```python
from build123d import *

# Parameters (mm, degrees)
F1_DEPTH = 50
F0_W     = 5
F0_H     = 13.255382
F2_DEPTH = 68
F3_R     = 2.6
F4_DEPTH = 9.584522
F5_R     = 5.083522
F6_DEPTH = 48


with BuildPart() as f1:
    # F0 (on Top) → F1 (new body)
    with BuildSketch(Plane.XY):
        with BuildLine():
            ThreePointArc((2.5, -6.627691), (5.826023, -4.029111), (7.083522, 0))
            ThreePointArc((7.083522, 0), (5.826023, 4.029111), (2.5, 6.627691))
            Line((2.5, 6.627691), (2.5, -6.627691))
        make_face()
        with BuildLine():
            Line((-2.5, 6.627691), (2.5, 6.627691))
            ThreePointArc((2.5, 6.627691), (0, 7.083522), (-2.5, 6.627691))
        make_face()
        with BuildLine():
            ThreePointArc((-2.5, -6.627691), (0, -7.083522), (2.5, -6.627691))
            Line((2.5, -6.627691), (-2.5, -6.627691))
        make_face()
        with BuildLine():
            Line((-2.5, -6.627691), (-2.5, 6.627691))
            ThreePointArc((-2.5, 6.627691), (-7.083522, 0), (-2.5, -6.627691))
        make_face()
    extrude(amount=F1_DEPTH)

    # F0 (on Top) → F2 (join)
    with BuildSketch(Plane.XY):
        Rectangle(F0_W, F0_H)
    extrude(amount=F2_DEPTH)

    # F3 (on face) → F4 (cut, through all)
    with BuildSketch(Plane.YZ.offset(2.5)):
        with Locations((0, 60)):
            Circle(F3_R)
    extrude(amount=-F4_DEPTH, mode=Mode.SUBTRACT)

    # F5 (on face) → F6 (cut)
    with BuildSketch(Plane(origin=(0, 0, 0), x_dir=(1, 0, 0), z_dir=(0, 0, -1))):
        Circle(F5_R)
    extrude(amount=-F6_DEPTH, mode=Mode.SUBTRACT)


solid = f1.part
```
Design review of the part built by this model. Coordinates are the model's own, in mm. A direction names the side the tool comes from. Give positions to 0.01 mm unless a question says otherwise; leave off trailing zeros. Loops run counter-clockwise (first coordinate to the right, second up) from the corner with the lowest first, then second, coordinate; pieces in that order, holes last. Notation, with made-up numbers: M -33.75,1.25 L -19.75,1.25 A30 ccw -19.75,24.25 Z; hole C 52.5,-28.75 d7. An arc over 180 degrees is marked long. Return JSON: item names as keys, results as strings. Group by question number.
Item 1: Insertion check: pin 1 Ø1.4 at (x, y) = (4.5, 0) entering from +Z; pin 2 Ø4 at (y, z) = (3, 48.5) entering from -X; pin 3 Ø5 at (x, z) = (-4.5, 44) entering from -Y. Each pin has a flat end and moves straight along its axis. Give the tip position at first contact, or say it passes through.
Item 2: We need section D-D (x = 4). Give the boundary of the cut face in (y, z).
Item 3: We need section B-B (x = -0.25). Give the boundary of the cut face in (y, z).
Item 4: For probe 1 along Y at (x, z) = (0, 37); probe 2 along X at (y, z) = (-2, 64), list the stretches that pass through material, from the lowest coordinate up.
Item 5: We need section C-C (z = 6). Give the boundary of the cut face in (x, y).
Item 6: We need section A-A (z = 60). Give the boundary of the cut face in (x, y).
Item 7: Mouldability with a two-part tool opening along Y and no side actions: class faces 1 (the flat face through (0, 6.628, 59)), 2 (the flat face through (-4, 0, 50)), 3 (the cylindrical face through (-1.102, 4.963, 23.664)), 4 (the cylindrical face through (0.04, 1.4, 62.19)) as released by +Y, released by -Y, zero draft, split by the parting line, or undercut.
Item 8: Tool access review of faces 5 (the flat face through (2.5, 0, 57)), 6 (the flat face through (0, 0, 68)), 7 (the flat face through (-2.5, 0, 57)), 8 (the flat face through (0, -6.628, 59)), 9 (the flat face through (0, 0, 48)): name each direction out of +Z, -Z, +X, -X, +Y, -Y from which nothing blocks a thin tool from reaching the whole face with its end or side.
Output:
{
 "1": {"pin 1": "stops at z = 50", "pin 2": "stops at x = -7.01", "pin 3": "stops at y = -6.8"},
 "2": {"outline": "M -5.85,0 L -3.14,0 L -3.14,48 L 3.14,48 L 3.14,0 L 5.85,0 L 5.85,50 L -5.85,50 Z"},
 "3": {"outline": "M -7.08,0 L -5.08,0 L -5.08,48 L 5.08,48 L 5.08,0 L 7.08,0 L 7.08,50 L 6.63,50 L 6.63,68 L -6.63,68 L -6.63,50 L -7.08,50 Z; hole C 0,60 d5.2"},
 "4": {"probe 1": "y = -7.08 to -5.08, 5.08 to 7.08", "probe 2": "x = -2.5 to 2.5"},
 "5": {"outline": "M -2.5,-6.63 A7.08 ccw 2.5,-6.63 A7.08 ccw 7.08,0 A7.08 ccw 2.5,6.63 A7.08 ccw -2.5,6.63 A7.08 ccw Z; hole C 0,0 d10.17"},
 "6": {"outline": "M -2.5,-6.63 L 2.5,-6.63 L 2.5,-2.6 L -2.5,-2.6 Z; M -2.5,2.6 L 2.5,2.6 L 2.5,6.63 L -2.5,6.63 Z"},
 "7": {"face 1": "released by +Y", "face 2": "zero draft", "face 3": "undercut", "face 4": "undercut"},
 "8": {"face 5": "+Z, +X, +Y, -Y", "face 6": "+Z, +X, -X, +Y, -Y", "face 7": "+Z, -X, +Y, -Y", "face 8": "+Z, +X, -X, -Y", "face 9": "-Z"}
}
